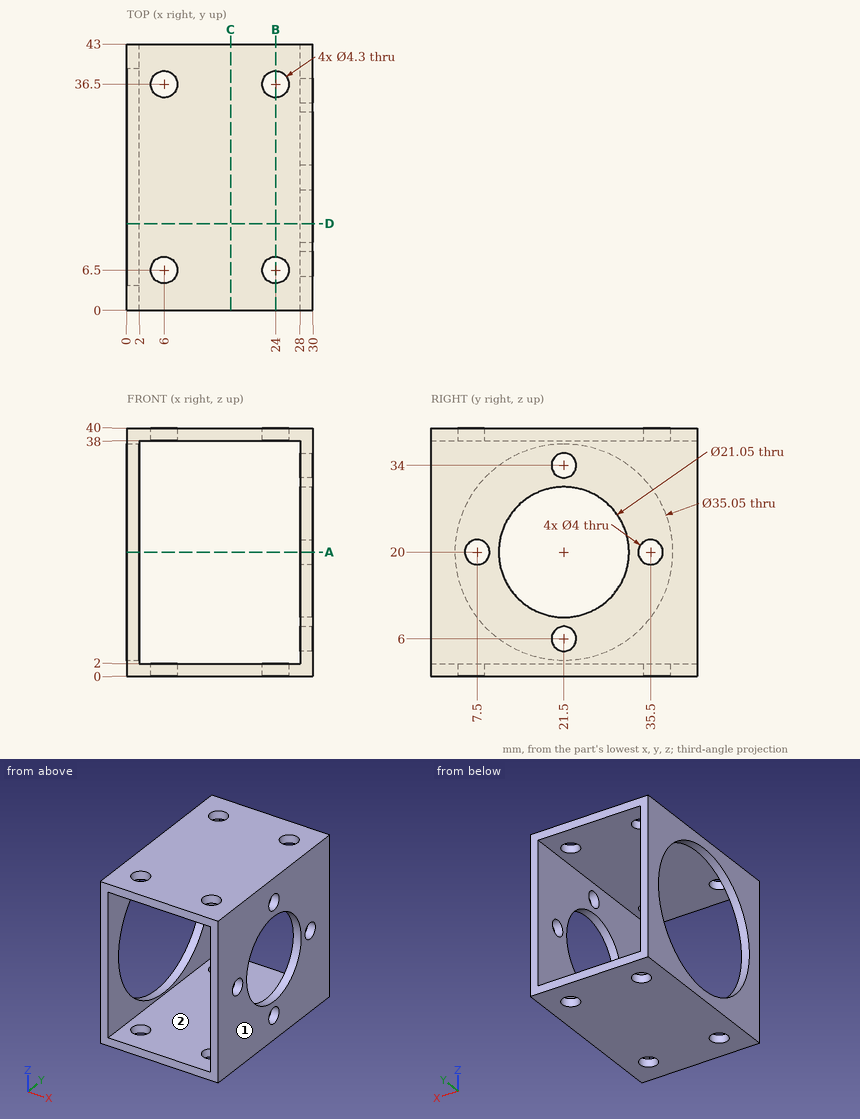
Source: three-view drawing plus pictorial views. Frame: mm from the lowest corner of the part. A direction names the side the tool comes from. Round coordinates to 2 decimals unless told otherwise and drop trailing zeros. Loops run counter-clockwise (first coordinate to the right, second up) from the corner with the lowest first, then second, coordinate; pieces in that order, holes last.
Q1. Section B-B on x = 24. Return loops of the section in (y, z).
Q2. Access query for the marked faces 1 and 2. Directions: +Z, -Z, +X, -X, +Y, -Y. A direction counts if a zero-diameter tool reaches every point of the face in a straight line with its end or side. Return the directions, or none.
Q3. Section C-C on x = 16.75. Return loops of the section in (y, z), plus the area to 3 significant figures.
Q4. Pin query (flat end, axial travel): P1, Ø2, axis at y = 28.5, z = 13, coming from the -X side. Return the tip coordinate at first contact, or that it passes through.
Q5. Section A-A on z = 20. Return loops of the section in (x, y) (3 decimals), plus the area to 3 significant figures.
Q6. Section D-D on y = 14. Return loops of the section in (x, z), plus the area to 3 significant figures.
Q7. Material intervals for L1, parallel to Y at x = 24, z = 39.6; L2, parallel to Z at x = 23, y = 15; L3, parallel to X at y = 2, z = 10, sorted ascending.
Evaluation:
1. outline: (0, 0) - (4.35, 0) - (4.35, 2) - (0, 2) - close; (0, 38) - (4.35, 38) - (4.35, 40) - (0, 40) - close; (8.65, 0) - (34.35, 0) - (34.35, 2) - (8.65, 2) - close; (8.65, 38) - (34.35, 38) - (34.35, 40) - (8.65, 40) - close; (38.65, 0) - (43, 0) - (43, 2) - (38.65, 2) - close; (38.65, 38) - (43, 38) - (43, 40) - (38.65, 40) - close
2. face 1: +Z, -Z, +X, +Y, -Y
2. face 2: +Y, -Y
3. outline: (0, 0) - (43, 0) - (43, 2) - (0, 2) - close; (0, 38) - (43, 38) - (43, 40) - (0, 40) - close
3. area: 172 mm2
4. P1: stops at x = 28
5. outline: (0, 0) - (2, 0) - (2, 3.975) - (0, 3.975) - close; (0, 39.025) - (2, 39.025) - (2, 43) - (0, 43) - close; (28, 0) - (30, 0) - (30, 5.5) - (28, 5.5) - close; (28, 9.5) - (30, 9.5) - (30, 10.975) - (28, 10.975) - close; (28, 32.025) - (30, 32.025) - (30, 33.5) - (28, 33.5) - close; (28, 37.5) - (30, 37.5) - (30, 43) - (28, 43) - close
5. area: 43.8 mm2
6. outline: (0, 0) - (30, 0) - (30, 12.62) - (28, 12.62) - (28, 2) - (2, 2) - (2, 4.16) - (0, 4.16) - close; (0, 35.84) - (2, 35.84) - (2, 38) - (28, 38) - (28, 27.38) - (30, 27.38) - (30, 40) - (0, 40) - close
6. area: 171 mm2
7. L1: y = 0 to 4.35, 8.65 to 34.35, 38.65 to 43
7. L2: z = 0 to 2, 38 to 40
7. L3: x = 0 to 2, 28 to 30
